Autodesk Inventor part; units mm, degrees
ref_plane "YZ Plane" through (0, 0, 0) normal (1, 0, 0) x (0, 1, 0)
ref_plane "XZ Plane" through (0, 0, 0) normal (0, 1, 0) x (-1, 0, 0)
ref_plane "XY Plane" through (0, 0, 0) normal (0, 0, 1) x (1, 0, 0)
sketch "Szkic1" plane through (0, 0, 0) normal (0, 1, 0) x (-1, 0, 0)
  line L0 (0, 0) -> (40, 0)
  line L1 (40, 0) -> (40, -20)
  line L2 (40, -20) -> (0, -20)
  line L3 (0, -20) -> (0, 0)
  dimension "d0" = 40
  dimension "d1" = 20
extrude "Wyciągnięcie proste1" add sketch "Szkic1" along normal blind 15
sketch "Szkic2" plane through (0, 15, 0) normal (0, 1, 0) x (1, 0, 0)
  line L0 (-40, 0) -> (0, 0) construction
  line L1 (0, 0) -> (0, 1.5) construction
  line L2 (0, 0) -> (0, 20) construction
  line L3 (0, 1.5) -> (-1.5, 1.5) construction
  line L4 (-1.5, 1.5) -> (-38.5, 1.5)
  line L5 (-38.5, 1.5) -> (-38.5, 18.5)
  line L6 (-38.5, 18.5) -> (-1.5, 18.5)
  line L7 (-1.5, 18.5) -> (-1.5, 1.5)
  dimension "d4" = 1.5
  dimension "d5" = 1.5
  dimension "d6" = 37
  dimension "d7" = 17
extrude "Wyciągnięcie proste2" cut sketch "Szkic2" against normal blind 12
sketch "Szkic3" plane through (-40, 0, 0) normal (0, 0, 1) x (1, 0, 0)
  line L0 (1.5, 3) -> (38.5, 3)
  line L1 (38.5, 15) -> (38.5, 3)
  line L2 (1.5, 3) -> (38.5, 3)
  line L3 (38.5, 3) -> (38.5, 15)
  line L4 (1.5, 15) -> (1.5, 3)
  line L5 (1.5, 15) -> (1.5, 3) construction
  line L6 (38.5, 15) -> (20, 15)
  line L7 (0, 15) -> (40, 15)
  line L8 (20, 15) -> (20, 10)
  line L9 (18, 9.5) -> (22, 9.5)
  line L10 (22, 9.5) -> (22, 10.5)
  line L11 (22, 10.5) -> (18, 10.5)
  line L12 (18, 10.5) -> (18, 9.5)
  line L13 (18, 9.5) -> (22, 10.5) construction
  line L14 (22, 9.5) -> (18, 10.5) construction
  point P0 (40, 0)
  dimension "d13" = 5
  dimension "d14" = 4
  dimension "d15" = 1
extrude "Wyciągnięcie proste3" add sketch "Szkic3" against normal blind 2.3 contours L11 L10 L9 L12
equation "\"d6\" = d0 - 2 * d5"
equation "\"d7\" = d1 - 2 * d5"
properties part number "obudowa_latarka_gora"
Build history of the part. All positions in model axes, mm. A direction names the side the tool comes from. Give positions to 0.01 mm unless a question says otherwise; leave off trailing zeros. Loops run counter-clockwise (first coordinate to the right, second up) from the corner with the lowest first, then second, coordinate; pieces in that order, holes last.
Item 1: Drill centre lines: line 1 (Z direction, x = -30.5, y = 11.75); line 2 (X direction, y = 10.5, z = -3.5); line 3 (Y direction, x = -25.5, z = -3.75). Where is each one in solid material? Low to high.
Answers follow:
line 1: z = -20 to -18.5, -1.5 to 0
line 2: x = -40 to -38.5, -1.5 to 0
line 3: y = 0 to 3
Item 2: Slice it at D-D, the plane x = -19.5. List the corners of the cut face in (y, z), and give its area (3 significant figures).
Answers follow:
outline: (0, -20) - (15, -20) - (15, -18.5) - (3, -18.5) - (3, -1.5) - (9.5, -1.5) - (9.5, -2.3) - (10.5, -2.3) - (10.5, -1.5) - (15, -1.5) - (15, 0) - (0, 0) - close
area: 96.8 mm2
Item 3: Slice it at A-A, the plane y = 5.75. List the corners of the cut face in (x, z), and give its area (3 significant figures).
Answers follow:
outline: (-40, -20) - (0, -20) - (0, 0) - (-40, 0) - close; hole (-38.5, -18.5) - (-1.5, -18.5) - (-1.5, -1.5) - (-38.5, -1.5) - close
area: 171 mm2
Item 4: Pull direction X, two halves, no side cores. Call faces 1 (the face through (-40, 7, -10)), 2 (the face through (-18, 15, -19)), 3 (the face through (-20, 9, -1.5)), 4 (the face through (0, 7, -10)): released by +X, released by -X, zero draft, split by the parting line, or undercut.
Answers follow:
face 1: released by -X
face 2: zero draft
face 3: undercut
face 4: released by +X
Item 5: Slice it at B-B, the plane z = -16.5. List the corners of the cut face in (x, y), and give its area (3 significant figures).
Answers follow:
outline: (-40, 0) - (0, 0) - (0, 15) - (-1.5, 15) - (-1.5, 3) - (-38.5, 3) - (-38.5, 15) - (-40, 15) - close
area: 156 mm2
Item 6: Which spindle directions (+Z, -Z, +X, -X, +Y, -Y) get a long thin tool onto all of the face, cutting with end or side? Do faces 5 (the face through (-20, 7, -20)), 6 (the face through (-38.5, 9, -10)). Say none if no direction does.
Answers follow:
face 5: -Z, +X, -X, +Y, -Y
face 6: +Y
Item 7: Flat gauge pin, fed straight in: pin 1 (1.5 mm diameter, centred on x = -16, z = -8, fed in from +Y). Where does the tip first touch, or does it go through?
Answers follow:
pin 1: stops at y = 3
Item 8: Slice it at C-C, the plane x = -27. List the corners of the cut face in (y, z).
Answers follow:
outline: (0, -20) - (15, -20) - (15, -18.5) - (3, -18.5) - (3, -1.5) - (15, -1.5) - (15, 0) - (0, 0) - close
